from build123d import *

# Parameters (mm, degrees)
CYLINDER001_R     = 7
CYLINDER001_DEPTH = 50
CYLINDER_R        = 8.5
CYLINDER_DEPTH    = 40
BOX_W             = 60
BOX_H             = 60
BOX_DEPTH         = 4
FILLET_R          = 8
FILLET001_R       = 2


with BuildPart() as cylinder001:
    # Cylinder001 → Cylinder001 (new body)
    with BuildSketch(Plane.XY):
        Circle(CYLINDER001_R)
    extrude(amount=CYLINDER001_DEPTH)


with BuildPart() as cylinder:
    # Cylinder → Cylinder (new body)
    with BuildSketch(Plane.XY):
        Circle(CYLINDER_R)
    extrude(amount=CYLINDER_DEPTH)


with BuildPart() as cut:
    # Box → Box (new body)
    with BuildSketch(Plane(origin=(-30, -30, 0), x_dir=(1, 0, 0), z_dir=(0, 0, 1))):
        with Locations((30, 30)):
            Rectangle(BOX_W, BOX_H)
    extrude(amount=BOX_DEPTH)

    # Fillet
    fillet_edges = [cut.edges().sort_by_distance(p)[0] for p in [
        (-30, -30, 2),
        (-30, 30, 2),
        (30, -30, 2),
        (30, 30, 2),
    ]]
    fillet(fillet_edges, radius=FILLET_R)

    # Fillet001
    fillet001_edges = [cut.edges().sort_by_distance(p)[0] for p in [
        (-30, 0, 4),
        (-27.656854, -27.656854, 4),
        (-27.656854, 27.656854, 4),
        (0, -30, 4),
        (0, 30, 4),
        (27.656854, -27.656854, 4),
        (27.656854, 27.656854, 4),
        (30, 0, 4),
    ]]
    fillet(fillet001_edges, radius=FILLET001_R)

    # Fusion: union Cylinder
    add(cylinder.part)

    # Cut: cut Cylinder001
    add(cylinder001.part, mode=Mode.SUBTRACT)


solid = cut.part
Work out the finished part from the listing and answer in its coordinate system (mm). A direction names the side the tool comes from. Coordinates: 2 decimals unless noted, no trailing zeros. Write each loop counter-clockwise with the first axis right and the second up, starting at its lowest first coordinate (ties: lowest second). Pieces come first, ordered by that corner, then holes. Notation, with made-up numbers: M 23,57.25 L 47,57.25 A28 cw 47,75.25 Z; hole C 87.25,-6 d8. An arc over 180 degrees is marked long. Write item = value, one per line.
1. Flat-ended cylindrical pins translate along their axes: pin 1 (12 mm diameter, centred on x = 4, z = 34.5, fed in from +Y); pin 2 (1 mm diameter, centred on x = -17, y = 7.5, fed in from -Z); pin 3 (12.5 mm diameter, centred on x = 0, y = 0, fed in from +Z); pin 4 (2 mm diameter, centred on y = -2.5, z = 31, fed in from -X). Find the tip coordinate at first contact, or state that the pin passes through.
Solution:
pin_1 = 8.5
pin_2 = 0
pin_3 = through
pin_4 = -8.37
2. The part is cut by section C-C (z = 22). Determine the outline of the cut face in (x, y).
Solution:
outline = C 0,0 d17; hole C 0,0 d14
3. Straight lines are drawn through the part: line 1 (X direction, y = 0, z = 29); line 2 (Z direction, x = -5, y = -9). For each, find the intervals that lie inside material, in ascending order. Write a range as from..to.
Solution:
line_1 = -8.5..-7, 7..8.5
line_2 = 0..4
4. The part is cut by section A-A (y = 0). Determine the outline of the cut face in (x, z), then the cut area to 3 significant figures.
Solution:
outline = M -30,0 L -7,0 L -7,40 L -8.5,40 L -8.5,4 L -28,4 A2 ccw -30,2 Z; M 7,0 L 30,0 L 30,2 A2 ccw 28,4 L 8.5,4 L 8.5,40 L 7,40 Z
area = 290 mm2
5. For faces 5 (the face through (0, -30, 1)), 6 (the face through (-7, 7, 4)), determine the directions among +Z, -Z, +X, -X, +Y, -Y from which every point of the face is accessible in a straight line to the end or side of a thin tool.
Solution:
face_5 = +Z, -Z, +X, -X, -Y
face_6 = +Z
6. Determine the mould class of faces 1 (the face through (-27.719, -27.594, 1.014)), 2 (the face through (29.43, -0.31, 3.4)), 3 (the face through (6.466, -2.681, 19.72)), 4 (the face through (0.31, 29.43, 3.4)) for opening direction X: released by +X, released by -X, zero draft, split by the parting line, or undercut.
Solution:
face_1 = released by -X
face_2 = released by +X
face_3 = undercut
face_4 = zero draft
7. The part is cut by section D-D (x = 16). Determine the outline of the cut face in (y, z).
Solution:
outline = M -30,0 L 30,0 L 30,2 A2 ccw 28,4 L -28,4 A2 ccw -30,2 Z
